Study the drawing (mm; zero at the part's minimum x, y, z) and answer. A direction names the side the tool comes from. Give positions to 0.01 mm unless a question says otherwise; leave off trailing zeros. Write each loop counter-clockwise with the first axis right and the second up, starting at its lowest first coordinate (ties: lowest second). Pieces come first, ordered by that corner, then holes. Notation, with made-up numbers: (-33.5, 26) - (-14.5, 26) arc R33 ccw to (-14.5, 57) - close; hole circle Ø10 at (73.5, -22.75). An arc over 180 degrees is marked (long way). One line per item, written item: value. Start each with the question number.
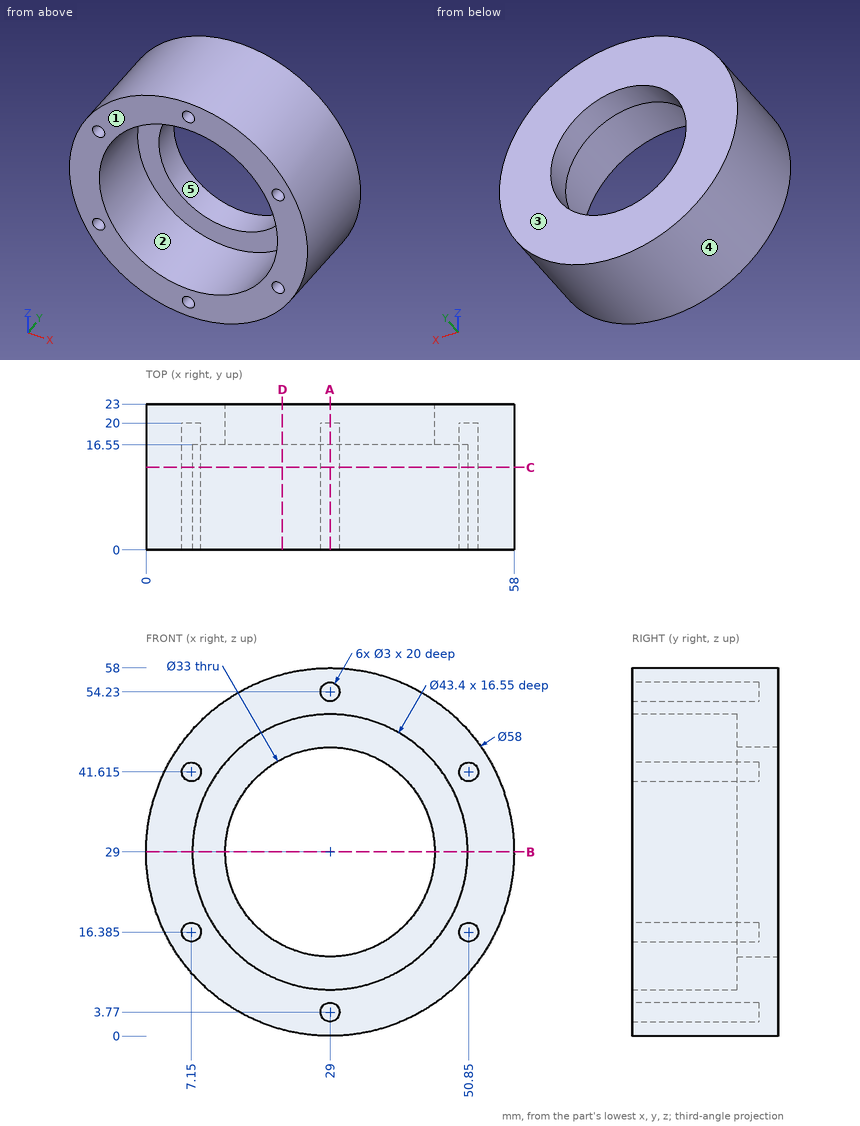
Item 1: Straight lines are drawn through the part: line 1 along X through (y, z) = (17.5, 41.5) (1 decimal); line 2 along X through (y, z) = (20.25, 29); line 3 along X through (y, z) = (4, 29). For each, find the intervals that lie inside material, in ascending order.
Item 2: Find section C-C on y = 13. Give the number of separate pieces and of enclosed holes in the cut face, plus the area to 3 significant figures.
Item 3: Find section B-B on z = 29. Determine the outline of the cut face in (x, y).
Item 4: Find section D-D on x = 21.5. Determine the outline of the cut face in (y, z), plus the area to 3 significant figures.
Item 5: For the marked faces 1 and 2, determine the directions among +Z, -Z, +X, -X, +Y, -Y from which every point of the face is accessible in a straight line to the end or side of a thin tool.
Item 6: The mould has two halves that part along X. Classify the marked faces 3, 4 and 5: +X half, -X half, draft (parallel to the pull), parting line (faces both ways), or undercut.
Item 7: Find section A-A on x = 29. Determine the outline of the cut face in (y, z), plus the area to 3 significant figures.
Item 8: Each of these flat-tipped pins is pushed along its axis until it touches: pin 1 Ø5 at (x, y) = (20.5, 15.5) entering from -Z; pin 2 Ø1 at (x, z) = (8.5, 51.5) entering from +Y; pin 3 Ø1 at (x, y) = (42, 11.5) entering from +Z; pin 4 Ø2.5 at (x, z) = (50.85, 16.38) entering from -Y. Where does it stop, or does it pass through?
Values:
1. line 1: 2.8 to 5.7, 8.6 to 18.2, 39.8 to 49.4, 52.3 to 55.2
1. line 2: 0 to 12.5, 45.5 to 58
1. line 3: 0 to 7.3, 50.7 to 58
2. separate pieces: 1
2. enclosed holes: 7
2. area: 1,120 mm^2
3. outline: (0, 0) - (7.3, 0) - (7.3, 16.55) - (12.5, 16.55) - (12.5, 23) - (0, 23) - close; (45.5, 16.55) - (50.7, 16.55) - (50.7, 0) - (58, 0) - (58, 23) - (45.5, 23) - close
4. outline: (0, 0.99) - (23, 0.99) - (23, 14.3) - (16.55, 14.3) - (16.55, 8.64) - (0, 8.64) - close; (0, 49.36) - (16.55, 49.36) - (16.55, 43.7) - (23, 43.7) - (23, 57.01) - (0, 57.01) - close
4. area: 425 mm^2
5. face 1: +Z, -Z, +X, -X, -Y
5. face 2: -Y
6. face 3: draft
6. face 4: parting line
6. face 5: undercut
7. outline: (0, 0) - (23, 0) - (23, 12.5) - (16.55, 12.5) - (16.55, 7.3) - (0, 7.3) - (0, 5.27) - (20, 5.27) - (20, 2.27) - (0, 2.27) - close; (0, 50.7) - (16.55, 50.7) - (16.55, 45.5) - (23, 45.5) - (23, 58) - (0, 58) - (0, 55.73) - (20, 55.73) - (20, 52.73) - (0, 52.73) - close
7. area: 283 mm^2
8. pin 1: z = 0.63
8. pin 2: through
8. pin 3: z = 55.17
8. pin 4: y = 20
